from build123d import *

# Parameters (mm, degrees)
EXTRUDE_THIN1_DEPTH = 120
SKETCH5_R           = 2
CUT_EXTRUDE1_DEPTH  = 145.568322948
FILLET1_R           = 1


with BuildPart() as part:
    # Sketch3 → Extrude-Thin1 (new body)
    with BuildSketch(Plane(origin=(0, 0, 0), x_dir=(0, 0, -1), z_dir=(1, 0, 0))):
        Polygon((-25, -30), (-25, 30), (25, 30), (25, -30), (35, -30), (35, 40), (-35, 40), (-35, -30), align=None)
    extrude(amount=EXTRUDE_THIN1_DEPTH)

    # Sketch5 → Cut-Extrude1 (cut, through all)
    with BuildSketch(Plane.XY.offset(35)):
        with Locations((26.536588231, -17.686450881)):
            Circle(SKETCH5_R)
        with Locations((93.76132228, -17.686450881)):
            Circle(SKETCH5_R)
    extrude(amount=-CUT_EXTRUDE1_DEPTH, mode=Mode.SUBTRACT)

    # Fillet1
    fillet1_edges = [part.edges().sort_by_distance(p)[0] for p in [
        (60, 40, 35),
        (60, 40, -35),
    ]]
    fillet(fillet1_edges, radius=FILLET1_R)


solid = part.part
Model file for the job. Use its own axes, mm. A direction names the side the tool comes from. Coordinates: 2 decimals unless noted, no trailing zeros. Write each loop counter-clockwise with the first axis right and the second up, starting at its lowest first coordinate (ties: lowest second). Pieces come first, ordered by that corner, then holes. Notation, with made-up numbers: (55, 55) -> (73, 55) arc R21 ccw to (73, 78) -> close; hole circle Ø6 at (32, 28.25). An arc over 180 degrees is marked (long way). One line per item, written item: value. Start each with the question number.
1) Probe probe 1 along Z at (x, y) = (81.5, 18.5); probe 2 along X at (y, z) = (-19, -28); probe 3 along Y at (x, z) = (38, 8.5). List the from-to ranges inside material, lowest first.
2) Flat gauge pins, fed straight in: pin 1 Ø10 at (y, z) = (28, -11.5) entering from -X; pin 2 Ø3 at (x, z) = (67, 7) entering from -Y. Where does each tip first touch, or does it go through?
3) Slice it at B-B on x = 89. Write the cut outline in (y, z), then the cut area to 3 significant figures.
4) Slice it at A-A on y = 22.5. Write the cut outline in (x, z).
5) Slice it at C-C on z = -9.5. Write the cut outline in (x, y), then the cut area to 3 significant figures.
6) Which spindle directions (+Z, -Z, +X, -X, +Y, -Y) get a long thin tool onto all of the face, cutting with end or side? Do faces 4 (the face through (59, 0, -25)), 5 (the face through (59, 40, 0)). Say none if no direction does.
7) Pull direction X, two halves, no side cores. Call faces 1 (the face through (120, 31, 3)), 2 (the face through (94.684, -19.461, 30.07)), 3 (the face through (59, 30, 0)): +X half, -X half, draft (parallel to the pull), parting line (faces both ways), or undercut.
Answers follow:
1. probe 1: -35 to -25, 25 to 35
1. probe 2: 0 to 25.03, 28.04 to 92.25, 95.27 to 120
1. probe 3: 30 to 40
2. pin 1: x = 0
2. pin 2: y = 30
3. outline: (-30, -35) -> (39, -35) arc R1 ccw to (40, -34) -> (40, 34) arc R1 ccw to (39, 35) -> (-30, 35) -> (-30, 25) -> (30, 25) -> (30, -25) -> (-30, -25) -> close
3. area: 1,900 mm2
4. outline: (0, -35) -> (120, -35) -> (120, -25) -> (0, -25) -> close; (0, 25) -> (120, 25) -> (120, 35) -> (0, 35) -> close
5. outline: (0, 30) -> (120, 30) -> (120, 40) -> (0, 40) -> close
5. area: 1,200 mm2
6. face 4: +X, -X, -Y
6. face 5: +Z, -Z, +X, -X, +Y
7. face 1: +X half
7. face 2: undercut
7. face 3: draft
